For this review, take the finished solid that the model builds, in its own axes (mm). Coordinates: 2 decimals unless noted, no trailing zeros. Loops run counter-clockwise (first coordinate to the right, second up) from the corner with the lowest first, then second, coordinate; pieces in that order, holes last.
1. Take a section at C-C, the plane x = 81. State the section outline as (y, z) points, then the cut area to 3 significant figures.
2. Take a section at B-B, the plane y = 60.5. State the section outline as (x, z) points.
3. Take a section at A-A, the plane z = 0.55. State the section outline as (x, y) points (1 decimal).
4. To check wall thickness, follow probe 1 along Y at (x, z) = (34, 0.5); probe 2 along Y at (x, z) = (-82, 0.25); probe 3 along X at (y, z) = (25, 1.5). State the ranges of each line that lie inside material, in increasing order.
5. Clearance check with a flat-ended pin moving along its axis: P1, Ø4, axis at x = 96.24, y = 55.56, coming from the -Z side. State where the tip first meets the part, or that it passes through.
```python
from build123d import *

# Parameters (mm, degrees)
SKETCH1_R             = 114.3
BOSS_EXTRUDE1_DEPTH   = 1.5875
F_4_CLEARANCE_HOLE1_D = 3.2639


with BuildPart() as part:
    # Sketch1 → Boss-Extrude1 (new body)
    with BuildSketch(Plane.XY):
        Circle(SKETCH1_R)
    extrude(amount=BOSS_EXTRUDE1_DEPTH)

    # #4 Clearance Hole1 (through all)
    with Locations(Plane(origin=(0, 111.125, 1.5875), x_dir=(1, 0, 0), z_dir=(0, 0, 1))):
        with Locations((0, 0), (96.237072996, -55.5625), (96.237072996, -166.6875), (0, -222.25), (-96.237072996, -166.6875), (-96.237072996, -55.5625)):
            Hole(F_4_CLEARANCE_HOLE1_D / 2)


solid = part.part
```
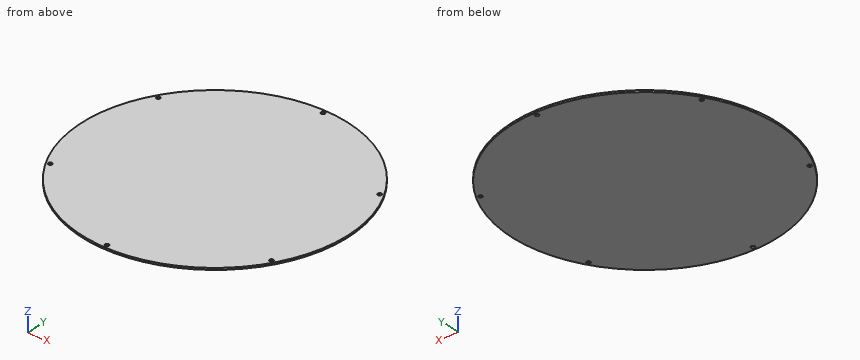
Results list:
1. outline: (-80.64, 0) - (80.64, 0) - (80.64, 1.59) - (-80.64, 1.59) - close
1. area: 256 mm2
2. outline: (-96.98, 0) - (96.98, 0) - (96.98, 1.59) - (-96.98, 1.59) - close
3. outline: circle Ø228.6 at (0, 0); hole circle Ø3.3 at (-96.2, -55.6); hole circle Ø3.3 at (-96.2, 55.6); hole circle Ø3.3 at (0, -111.1); hole circle Ø3.3 at (0, 111.1); hole circle Ø3.3 at (96.2, -55.6); hole circle Ø3.3 at (96.2, 55.6)
4. probe 1: y = -109.13 to 109.13
4. probe 2: y = -79.63 to 79.63
4. probe 3: x = -111.53 to 111.53
5. P1: stops at z = 0
